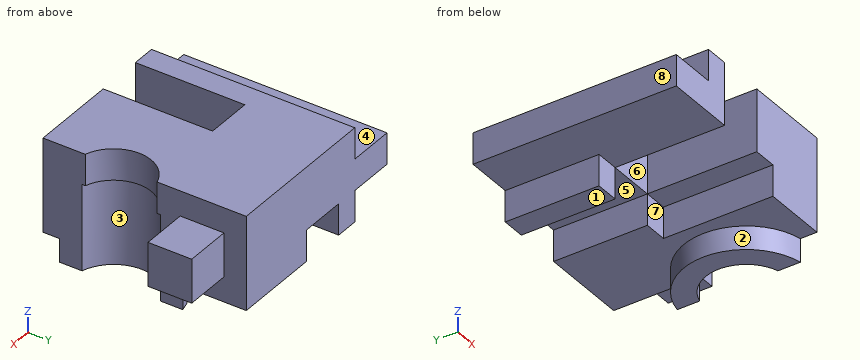
```python
from build123d import *

# Parameters (mm, degrees)
SKETCH1_R            = 1
BOSS_EXTRUDE1_DEPTH  = 6
SKETCH2_R            = 2.6
CUT_EXTRUDE1_DEPTH   = 6
SKETCH3_W            = 7.6
SKETCH3_H            = 13
BOSS_EXTRUDE2_DEPTH  = 6
BOSS_EXTRUDE5_START  = -5
SKETCH6_W            = 3
SKETCH6_H            = 2
BOSS_EXTRUDE5_DEPTH  = 13
BOSS_EXTRUDE6_START  = -7.5
SKETCH10_R           = 4
SKETCH10_R_2         = 2.6
BOSS_EXTRUDE6_DEPTH  = 1.5
BOSS_EXTRUDE7_START  = -6
SKETCH12_R           = 2.6
SKETCH12_R_2         = 2.4
BOSS_EXTRUDE7_DEPTH  = 2
CUT_EXTRUDE2_DEPTH   = 7
SKETCH14_W           = 3
SKETCH14_H           = 6
CUT_EXTRUDE3_DEPTH   = 2
SKETCH15_W           = 0.2
SKETCH15_H           = 13
CUT_EXTRUDE5_DEPTH   = 7.5
SKETCH16_W           = 3
SKETCH16_H           = 3
CUT_EXTRUDE6_DEPTH   = 3
SKETCH17_W           = 2.8
SKETCH17_H           = 2.8
BOSS_EXTRUDE9_DEPTH  = 3
BOSS_EXTRUDE10_START = 24.4
SKETCH17_2_W         = 2.8
SKETCH17_2_H         = 2.8
BOSS_EXTRUDE10_DEPTH = 3
SKETCH18_W           = 29.7
SKETCH18_H           = 13
CUT_EXTRUDE11_DEPTH  = 9
SKETCH21_W           = 2.8
SKETCH21_H           = 2.8
BOSS_EXTRUDE12_DEPTH = 3


with BuildPart() as part:
    # Sketch1 → Boss-Extrude1 (new body)
    with BuildSketch(Plane.XY):
        with BuildLine():
            ThreePointArc((3.75, -5), (4.47902769, -4.358991965), (5.1, -3.61282438))
            Line((5.1, -3.61282438), (5.1, 3.61282438))
            ThreePointArc((5.1, 3.61282438), (0, 6.25), (-5.1, 3.61282438))
            Line((-5.1, 3.61282438), (-5.1, -3.61282438))
            ThreePointArc((-5.1, -3.61282438), (-4.47902769, -4.358991965), (-3.75, -5))
            Line((-3.75, -5), (-14.7, -5))
            Line((-14.7, -5), (-14.7, 8))
            Line((-14.7, 8), (14.7, 8))
            Line((14.7, 8), (14.7, -5))
            Line((14.7, -5), (3.75, -5))
        make_face()
        with Locations((11.5, 0)):
            Circle(SKETCH1_R, mode=Mode.SUBTRACT)
        with Locations((-11.5, 0)):
            Circle(SKETCH1_R, mode=Mode.SUBTRACT)
    extrude(amount=BOSS_EXTRUDE1_DEPTH)

    # Sketch2 → Cut-Extrude1 (cut)
    with BuildSketch(Plane.XY):
        with Locations((-11.5, 0)):
            Circle(SKETCH2_R)
        with Locations((11.5, 0)):
            Circle(SKETCH2_R)
    extrude(amount=CUT_EXTRUDE1_DEPTH, mode=Mode.SUBTRACT)

    # Sketch3 → Boss-Extrude2 (add)
    with BuildSketch(Plane.XY):
        with Locations((-18.5, 1.5)):
            Rectangle(SKETCH3_W, SKETCH3_H)
    extrude(amount=BOSS_EXTRUDE2_DEPTH)

    # Sketch6 → Boss-Extrude5 (add)
    with BuildSketch(Plane(origin=(0, 0, 0), x_dir=(1, 0, 0), z_dir=(0, 1, 0)).offset(BOSS_EXTRUDE5_START)):
        with Locations((-23.8, -3)):
            Rectangle(SKETCH6_W, SKETCH6_H)
        with Locations((16.2, -3)):
            Rectangle(SKETCH6_W, SKETCH6_H)
    extrude(amount=BOSS_EXTRUDE5_DEPTH)

    # Sketch10 → Boss-Extrude6 (add)
    with BuildSketch(Plane.XY.offset(6).offset(BOSS_EXTRUDE6_START)):
        with Locations((-11.5, 0)):
            Circle(SKETCH10_R)
        with Locations((-11.5, 0)):
            Circle(SKETCH10_R_2, mode=Mode.SUBTRACT)
        with BuildLine():
            Line((14.7, 2.4), (14.7, -2.4))
            ThreePointArc((14.7, -2.4), (7.5, 0), (14.7, 2.4))
        make_face()
        with Locations((11.5, 0)):
            Circle(SKETCH10_R_2, mode=Mode.SUBTRACT)
    extrude(amount=BOSS_EXTRUDE6_DEPTH)

    # Sketch12 → Boss-Extrude7 (add)
    with BuildSketch(Plane(origin=(0, 0, 0), x_dir=(-1, 0, 0), z_dir=(0, 0, -1)).offset(BOSS_EXTRUDE7_START)):
        with Locations((11.5, 0)):
            Circle(SKETCH12_R)
        with Locations((11.5, 0)):
            Circle(SKETCH12_R_2, mode=Mode.SUBTRACT)
        with Locations((-11.5, 0)):
            Circle(SKETCH12_R)
        with Locations((-11.5, 0)):
            Circle(SKETCH12_R_2, mode=Mode.SUBTRACT)
    extrude(amount=BOSS_EXTRUDE7_DEPTH)

    # Sketch13 → Cut-Extrude2 (cut)
    with BuildSketch(Plane.XZ.offset(5)):
        Polygon((-22.3, 0), (-16.3, 0), (-16.3, 2), (-17.8, 2), (-17.8, 6), (-20.8, 6), (-20.8, 2), (-22.3, 2), align=None)
    extrude(amount=-CUT_EXTRUDE2_DEPTH, mode=Mode.SUBTRACT)

    # Sketch14 → Cut-Extrude3 (cut)
    with BuildSketch(Plane(origin=(0, 0, 0), x_dir=(-1, 0, 0), z_dir=(0, 0, -1))):
        with Locations((19.3, 5)):
            Rectangle(SKETCH14_W, SKETCH14_H)
    extrude(amount=-CUT_EXTRUDE3_DEPTH, mode=Mode.SUBTRACT)

    # Sketch15 → Cut-Extrude5 (cut, symmetric)
    with BuildSketch(Plane.XY):
        with Locations((-12.1, 1.5)):
            Rectangle(SKETCH15_W, SKETCH15_H)
        with Locations((12.1, 1.5)):
            Rectangle(SKETCH15_W, SKETCH15_H)
    extrude(amount=CUT_EXTRUDE5_DEPTH, both=True, mode=Mode.SUBTRACT)

    # Sketch16 → Cut-Extrude6 (cut)
    with BuildSketch(Plane(origin=(12, 0, 0), x_dir=(0, 0, -1), z_dir=(1, 0, 0))):
        with Locations((-3, 5.173669459)):
            Rectangle(SKETCH16_W, SKETCH16_H)
    cut_extrude6 = extrude(amount=-CUT_EXTRUDE6_DEPTH, mode=Mode.SUBTRACT)

    # Mirror1: Cut-Extrude6 across plane
    add(cut_extrude6.mirror(Plane(origin=(0, 0, 0), x_dir=(0, 0, 1), z_dir=(1, 0, 0))), mode=Mode.SUBTRACT)

    # Sketch17 → Boss-Extrude9 (add)
    with BuildSketch(Plane(origin=(-12.2, 0, 0), x_dir=(0, 0, -1), z_dir=(1, 0, 0))):
        with Locations((-3, 5.173669459)):
            Rectangle(SKETCH17_W, SKETCH17_H)
    extrude(amount=BOSS_EXTRUDE9_DEPTH)

    # Sketch17<2> → Boss-Extrude10 (add)
    with BuildSketch(Plane(origin=(-12.2, 0, 0), x_dir=(0, 0, -1), z_dir=(1, 0, 0)).offset(BOSS_EXTRUDE10_START)):
        with Locations((-3, 5.173669459)):
            Rectangle(SKETCH17_2_W, SKETCH17_2_H)
    extrude(amount=-BOSS_EXTRUDE10_DEPTH)

    # Sketch18 → Cut-Extrude11 (cut, symmetric)
    with BuildSketch(Plane.XY):
        with Locations((2.85, 1.5)):
            Rectangle(SKETCH18_W, SKETCH18_H)
    extrude(amount=CUT_EXTRUDE11_DEPTH, both=True, mode=Mode.SUBTRACT)

    # Sketch21 → Boss-Extrude12 (add)
    with BuildSketch(Plane(origin=(-12.2, 0, 0), x_dir=(0, 0, -1), z_dir=(1, 0, 0))):
        with Locations((-3, 5.173669459)):
            Rectangle(SKETCH21_W, SKETCH21_H)
    extrude(amount=BOSS_EXTRUDE12_DEPTH)


solid = part.part
```
The listing builds one solid part. Answer for the finished solid, in the listing's coordinates (mm). Face numbers are marked on the shaded views. A direction names the side the tool comes from. Coordinates: 2 decimals unless noted, no trailing zeros. Write each loop counter-clockwise with the first axis right and the second up, starting at its lowest first coordinate (ties: lowest second). Pieces come first, ordered by that corner, then holes. Notation, with made-up numbers: (49, 62) - (64, 62) arc R17 ccw to (64, 79) - close; hole circle Ø3 at (24.5, -14.75). An arc over 180 degrees is marked (long way). One line per item, written item: value.
1) Find section B-B (y = 0.75). Give the vertices of the cut face in (x, z), and give its area (3 significant figures).
Geometry check:
outline: (-25.3, 2) - (-20.8, 2) - (-20.8, 6) - (-22.3, 6) - (-22.3, 4) - (-25.3, 4) - close; (-17.8, 2) - (-16.3, 2) - (-16.3, 0) - (-15.43, 0) - (-15.43, -1.5) - (-13.99, -1.5) - (-13.99, 4) - (-13.78, 4) - (-13.78, 6) - (-17.8, 6) - close
area: 34.4 mm2
2) A tool of negligible diameter and unlimited length cuts with its end or side. For the marked faces 1, 2, 3, 4 and 5, from which of +Z, -Z, +X, -X, +Y, -Y can it reach the whole face along a straight path? Write none if from no direction.
Geometry check:
face 1: -Z, -X, +Y, -Y
face 2: -Z, -X
face 3: -Z, +X
face 4: +Z, -X, +Y, -Y
face 5: -Z, +Y, -Y
3) For a pull along X with two mould halves and no side action, classify the marked faces 6, 7 and 8 as pulls with the +X half, pulls with the -X half, needs draft (parallel to the pull), parting line crosses it, or undercut.
Geometry check:
face 6: undercut
face 7: needs draft
face 8: pulls with the -X half
4) Consider line 1 along Z through (x, y) = (-12, 5.75); line 2 along Z through (x, y) = (-22, 2.5); line 3 along Y through (x, z) = (-20, 2.75). Determine where each line is inside the solid, lowest interval first. Write a range as from..to.
Geometry check:
line 1: z = 1.6..4.4
line 2: z = 0..6
line 3: y = 2..8
5) Find section A-A (z = 1.25). Give the vertices of the cut face in (x, y), and give its area (3 significant figures).
Geometry check:
outline: (-22.3, 2) - (-20.8, 2) - (-20.8, 8) - (-22.3, 8) - close; (-17.8, 2) - (-16.3, 2) - (-16.3, -5) - (-12.2, -5) - (-12.2, -2.5) arc R2.6 cw to (-12.2, 2.5) - (-12.2, 8) - (-17.8, 8) - close
area: 64.3 mm2
6) Find section C-C (z = 5). Give the vertices of the cut face in (x, y).
Geometry check:
outline: (-22.3, -5) - (-20.8, -5) - (-20.8, 2) - (-17.8, 2) - (-17.8, -5) - (-12.2, -5) - (-12.2, -2.3) arc R2.4 cw to (-12.2, 2.3) - (-12.2, 8) - (-22.3, 8) - close
7) Find section D-D (x = -22). Give the vertices of the cut face in (y, z).
Geometry check:
outline: (-5, 2) - (2, 2) - (2, 0) - (8, 0) - (8, 6) - (-5, 6) - close
8) Each of these flat-tipped pins is pushed along its axis until it touches: pin 1 Ø0.9 at (x, y) = (-23.5, 4.5) entering from +Z; pin 2 Ø1.2 at (x, z) = (-17, 1) entering from -Y; pin 3 Ø0.9 at (x, y) = (-19, 6.5) entering from -Z. Where does it stop, or does it pass through?
Geometry check:
pin 1: stops at z = 4
pin 2: stops at y = 2
pin 3: stops at z = 2
